Read the model definition and answer for the solid it produces. Units are mm, in the model's axes. A direction names the side the tool comes from. Round coordinates to 2 decimals unless told otherwise and drop trailing zeros. Loops run counter-clockwise (first coordinate to the right, second up) from the corner with the lowest first, then second, coordinate; pieces in that order, holes last. Notation, with made-up numbers: M 79,-33.75 L 127,-33.75 A4 ccw 127,-29.75 Z; hole C 78.25,81 d11. An arc over 180 degrees is marked long. Write each question's results on one line, items separated by ' | '.
from build123d import *

# Parameters (mm, degrees)
SKETCH1_W                = 30
SKETCH1_H                = 350
BOSS_EXTRUDE1_DEPTH      = 30
BOSS_EXTRUDE2_DEPTH      = 40
BOSS_EXTRUDE2_DEPTH_BACK = 70
SKETCH2_R                = 15


with BuildPart() as part:
    # Sketch1 → Boss-Extrude1 (new body)
    with BuildSketch(Plane.XY):
        Rectangle(SKETCH1_W, SKETCH1_H)
    extrude(amount=BOSS_EXTRUDE1_DEPTH)

    # Sketch2 → Boss-Extrude2 (add, two sides: drawn at the far end of the back side and taken through both)
    with BuildSketch(Plane(origin=(15, 0, 0), x_dir=(0, 0, -1), z_dir=(1, 0, 0)).offset(-BOSS_EXTRUDE2_DEPTH_BACK)):
        with Locations(Location((-15, -175, 0), (0, 0, 90))):
            Circle(SKETCH2_R)
    extrude(amount=BOSS_EXTRUDE2_DEPTH + BOSS_EXTRUDE2_DEPTH_BACK)

    # Mirror1: part across plane


with BuildPart() as part_1:
    add(part.part)
    add(part.part.mirror(Plane(origin=(-15, 175, 30), x_dir=(0, 0, 1), z_dir=(0, -1, 0))))


solid = part_1.part
Item 1: The part is cut by section A-A (z = 15). Determine the outline of the cut face in (x, y).
Outcome:
outline: M -55,-190 L 55,-190 L 55,-160 L 15,-160 L 15,510 L 55,510 L 55,540 L -55,540 L -55,510 L -15,510 L -15,-160 L -55,-160 Z
Item 2: Straight lines are drawn through the part: line 1 (Y direction, x = -29, z = 13.75); line 2 (X direction, y = 177.5, z = 9.5); line 3 (Y direction, x = -42.5, z = 1.75). For each, find the intervals that lie inside material, in ascending order.
Outcome:
line 1: y = -189.95 to -160.05, 510.05 to 539.95 | line 2: x = -15 to 15 | line 3: y = -182.03 to -167.97, 517.97 to 532.03
Item 3: Flat-ended cylindrical pins translate along their axes: pin 1 (1 mm diameter, centred on y = 258.5, z = 25, fed in from -X); pin 2 (8 mm diameter, centred on x = 14.5, z = 19.5, fed in from -Y); pin 3 (15 mm diameter, centred on y = 178, z = 19, fed in from +X). Find the tip coordinate at first contact, or state that the pin passes through.
Outcome:
pin 1: stops at x = -15 | pin 2: stops at y = -189.99 | pin 3: stops at x = 15
Item 4: For faces 1 (the face through (-55, 525, 15)), 2 (the face through (-0.77, -189.985, 15.66)), determine the directions among +Z, -Z, +X, -X, +Y, -Y from which every point of the face is accessible in a straight line to the end or side of a thin tool.
Outcome:
face 1: +Z, -Z, -X, +Y, -Y | face 2: none
Item 5: The mould has two halves that part along Y. Classify faces 3 (the face through (0, 170, 30)), 4 (the face through (-0.77, 539.985, 15.66)): pulls with the +Y half, pulls with the -Y half, needs draft (parallel to the pull), parting line crosses it, or undercut.
Outcome:
face 3: needs draft | face 4: undercut
Item 6: The part is cut by section C-C (y = 143.5). Determine the outline of the cut face in (x, z).
Outcome:
outline: M -15,0 L 15,0 L 15,30 L -15,30 Z
Item 7: The part is cut by section B-B (x = -28.5). Determine the outline of the cut face in (y, z), plus the area to 3 significant figures.
Outcome:
outline: C -175,15 d30; C 525,15 d30 | area: 1,410 mm2
